Could you check a few things on this model? Use its own coordinates, in mm. Coordinates: 2 decimals unless noted, no trailing zeros. Order: outer loops, then holes, each group sorted by start corner. A loop starts at its lowest first (then second) coordinate and runs counter-clockwise, first axis right, second up. Notation, with made-up numbers: (82.25, -2.75) -> (91.25, -2.75) arc R19 cw to (91.25, 29.25) -> close; hole circle Ø4 at (6.5, 33.25). An arc over 180 degrees is marked (long way). Return JSON: item names as keys, results as strings. Group by question number.
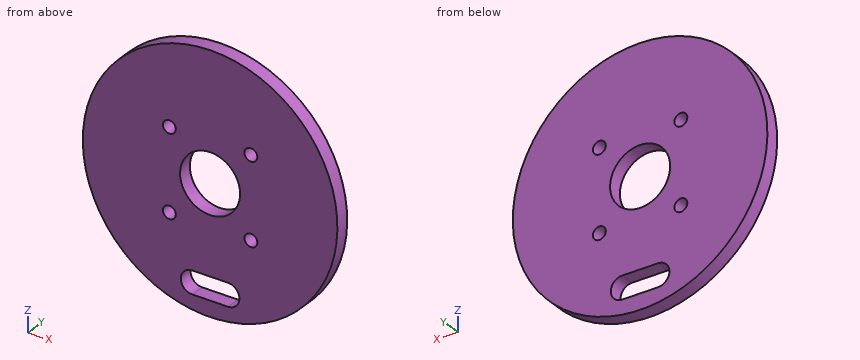
from build123d import *

# Parameters (mm, degrees)
SKETCH1_R            = 44.5
SKETCH1_R_2          = 10.5
BODY_DEPTH           = 5
WIRE_HOLE_DEPTH      = 64.130816564
M4_CLEARANCE_HOLE1_D = 4.5


with BuildPart() as part:
    # Sketch1 → Body (new body)
    with BuildSketch(Plane(origin=(0, 0, 0), x_dir=(1, 0, 0), z_dir=(0, 1, 0))):
        with Locations(Location((0, 0, 0), (0, 0, 270))):
            Circle(SKETCH1_R)
        with Locations(Location((0, 0, 0), (0, 0, 270))):
            Circle(SKETCH1_R_2, mode=Mode.SUBTRACT)
    extrude(amount=BODY_DEPTH)

    # Sketch5 → Wire_Hole (cut, through all)
    with BuildSketch(Plane(origin=(0, 5, 0), x_dir=(1, 0, 0), z_dir=(0, 1, 0))):
        with BuildLine():
            Line((-6.25, 39), (6.25, 39))
            ThreePointArc((6.25, 39), (10.25, 35), (6.25, 31))
            Line((6.25, 31), (-6.25, 31))
            ThreePointArc((-6.25, 31), (-10.25, 35), (-6.25, 39))
        make_face()
    extrude(amount=-WIRE_HOLE_DEPTH, mode=Mode.SUBTRACT)

    # M4 Clearance Hole1 (through all)
    with Locations(Plane(origin=(0, 5, 0), x_dir=(1, 0, 0), z_dir=(0, 1, 0))):
        with Locations((-14.25, 14.25), (14.25, -14.25), (14.25, 14.25), (-14.25, -14.25)):
            Hole(M4_CLEARANCE_HOLE1_D / 2)


solid = part.part
Q1. I'm going to push flat-ended pins straight in: pin 1 Ø2 at (x, y) = (-20, 1) entering from -Z; pin 2 Ø2 at (y, z) = (2, -1.5) entering from -X; pin 3 Ø2.5 at (x, y) = (1.5, 3) entering from +Z. Where does each tip first touch, or does it pass through?
Q2. I want a section at C-C on y = 1.65. Please give me the cut outline in (x, z).
Q3. I want a section at A-A on x = 0. Please give me the cut outline in (y, z).
Q4. I need wall thicknesses on line 1 along X through (y, z) = (3.9, 14.25); line 2 along Z through (x, y) = (12.5, 1.95). Which ranges of each line are inside material? Lowest first, please. Write a range as from..to.
Q5. I want a section at D-D on z = 7.5. Please give me the cut outline in (x, y), and give its area (3 significant figures).
Q6. I want a section at B-B on z = -14.25. Please give me the cut outline in (x, y), and give its area (3 significant figures).
Response values:
{
 "1": {"pin 1": "stops at z = -40.24", "pin 2": "stops at x = -44.5", "pin 3": "stops at z = 44.5"},
 "2": {"outline": "circle Ø89 at (0, 0); hole circle Ø4.5 at (-14.25, -14.25); hole circle Ø4.5 at (-14.25, 14.25); hole circle Ø21 at (0, 0); hole (-6.25, -39) -> (6.25, -39) arc R4 ccw to (6.25, -31) -> (-6.25, -31) arc R4 ccw to start; hole circle Ø4.5 at (14.25, -14.25); hole circle Ø4.5 at (14.25, 14.25)"},
 "3": {"outline": "(0, -44.5) -> (5, -44.5) -> (5, -39) -> (0, -39) -> close; (0, -31) -> (5, -31) -> (5, -10.5) -> (0, -10.5) -> close; (0, 10.5) -> (5, 10.5) -> (5, 44.5) -> (0, 44.5) -> close"},
 "4": {"line 1": "x = -42.16..-16.5, -12..12, 16.5..42.16", "line 2": "z = -42.71..-15.66, -12.84..12.84, 15.66..42.71"},
 "5": {"outline": "(-43.86, 0) -> (-7.35, 0) -> (-7.35, 5) -> (-43.86, 5) -> close; (7.35, 0) -> (43.86, 0) -> (43.86, 5) -> (7.35, 5) -> close", "area": "365 mm²"},
 "6": {"outline": "(-42.16, 0) -> (-16.5, 0) -> (-16.5, 5) -> (-42.16, 5) -> close; (-12, 0) -> (12, 0) -> (12, 5) -> (-12, 5) -> close; (16.5, 0) -> (42.16, 0) -> (42.16, 5) -> (16.5, 5) -> close", "area": "377 mm²"}
}
